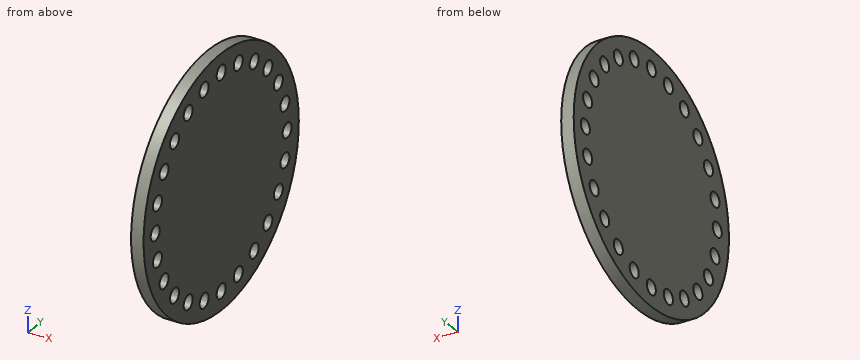
from build123d import *

# Parameters (mm, degrees)
F0_R     = 30
F0_R_2   = 1.75
F1_DEPTH = 3


with BuildPart() as f1:
    # F0 (on Right) → F1 (new body)
    with BuildSketch(Plane.YZ):
        Circle(F0_R)
        with Locations((-18.031223, -18.031223)):
            Circle(F0_R_2, mode=Mode.SUBTRACT)
        with Locations((-6.599886, -24.631109)):
            Circle(F0_R_2, mode=Mode.SUBTRACT)
        with Locations((-12.75, -22.083648)):
            Circle(F0_R_2, mode=Mode.SUBTRACT)
        with Locations((-22.083648, -12.75)):
            Circle(F0_R_2, mode=Mode.SUBTRACT)
        with Locations((-24.631109, -6.599886)):
            Circle(F0_R_2, mode=Mode.SUBTRACT)
        with Locations((0, -25.5)):
            Circle(F0_R_2, mode=Mode.SUBTRACT)
        with Locations((6.599886, -24.631109)):
            Circle(F0_R_2, mode=Mode.SUBTRACT)
        with Locations((12.75, -22.083648)):
            Circle(F0_R_2, mode=Mode.SUBTRACT)
        with Locations((18.031223, -18.031223)):
            Circle(F0_R_2, mode=Mode.SUBTRACT)
        with Locations((22.083648, -12.75)):
            Circle(F0_R_2, mode=Mode.SUBTRACT)
        with Locations((24.631109, -6.599886)):
            Circle(F0_R_2, mode=Mode.SUBTRACT)
        with Locations((-25.5, 0)):
            Circle(F0_R_2, mode=Mode.SUBTRACT)
        with Locations((-24.631109, 6.599886)):
            Circle(F0_R_2, mode=Mode.SUBTRACT)
        with Locations((-22.083648, 12.75)):
            Circle(F0_R_2, mode=Mode.SUBTRACT)
        with Locations((-18.031223, 18.031223)):
            Circle(F0_R_2, mode=Mode.SUBTRACT)
        with Locations((-12.75, 22.083648)):
            Circle(F0_R_2, mode=Mode.SUBTRACT)
        with Locations((-6.599886, 24.631109)):
            Circle(F0_R_2, mode=Mode.SUBTRACT)
        with Locations((25.5, 0)):
            Circle(F0_R_2, mode=Mode.SUBTRACT)
        with Locations((24.631109, 6.599886)):
            Circle(F0_R_2, mode=Mode.SUBTRACT)
        with Locations((22.083648, 12.75)):
            Circle(F0_R_2, mode=Mode.SUBTRACT)
        with Locations((12.75, 22.083648)):
            Circle(F0_R_2, mode=Mode.SUBTRACT)
        with Locations((0, 25.5)):
            Circle(F0_R_2, mode=Mode.SUBTRACT)
        with Locations((6.599886, 24.631109)):
            Circle(F0_R_2, mode=Mode.SUBTRACT)
        with Locations((18.031223, 18.031223)):
            Circle(F0_R_2, mode=Mode.SUBTRACT)
    extrude(amount=F1_DEPTH)


solid = f1.part
Check sheet for the modelled part. Datum: model origin and axes. Units: mm. Coordinates: 2 decimals unless noted, no trailing zeros. Loops run counter-clockwise (first coordinate to the right, second up) from the corner with the lowest first, then second, coordinate; pieces in that order, holes last. Notation, with made-up numbers: (22.25, 60) -> (73.25, 60) arc R17 ccw to (73.25, 93) -> close; hole circle Ø4 at (26, -7). An arc over 180 degrees is marked (long way). Answer in a Markdown table with one row per item.
1. Material ranges on line 1 along Z through (x, y) = (1.5, 0); line 2 along Y through (x, z) = (0.35, 12); line 3 along Y through (x, z) = (0.95, -24), recorded low to high. Write a range as [from, to].
Check values:
| item | result |
|---|---|
| line 1 | z = [-30, -27.25], [-23.75, 23.75], [27.25, 30] |
| line 2 | y = [-27.5, -23.66], [-20.5, 20.5], [23.66, 27.5] |
| line 3 | y = [-18, -8.23], [-4.97, -0.9], [0.9, 4.97], [8.23, 18] |
2. Sectioned sample at A-A, the plane z = 0. Record the boundary of the cut face in (x, y), then the cut area to 3 significant figures.
Check values:
| item | result |
|---|---|
| outline | (0, -30) -> (3, -30) -> (3, -27.25) -> (0, -27.25) -> close; (0, -23.75) -> (3, -23.75) -> (3, 23.75) -> (0, 23.75) -> close; (0, 27.25) -> (3, 27.25) -> (3, 30) -> (0, 30) -> close |
| area | 159 mm2 |
3. Sectioned sample at D-D, the plane y = -25.5. Record the boundary of the cut face in (x, z), then the cut area to 3 significant figures.
Check values:
| item | result |
|---|---|
| outline | (0, -15.8) -> (3, -15.8) -> (3, -8.12) -> (0, -8.12) -> close; (0, -5.08) -> (3, -5.08) -> (3, -1.75) -> (0, -1.75) -> close; (0, 1.75) -> (3, 1.75) -> (3, 5.08) -> (0, 5.08) -> close; (0, 8.12) -> (3, 8.12) -> (3, 15.8) -> (0, 15.8) -> close |
| area | 66.1 mm2 |
4. Sectioned sample at C-C, the plane x = 1.95. Give the number of separate pieces and of enclosed holes in the cut face, then the cut area to 3 significant figures.
Check values:
| item | result |
|---|---|
| separate pieces | 1 |
| enclosed holes | 24 |
| area | 2,600 mm2 |
5. Go/stop test with flat-tipped pins: pin 1 (1 mm diameter, centred on x = 1.5, y = 16, fed in from +Z); pin 2 (3 mm diameter, centred on y = -18.03, z = -18.03, fed in from +X); pin 3 (1 mm diameter, centred on x = 2, y = 20.5, fed in from -Z). Record where each tip stops, or that it passes through.
Check values:
| item | result |
|---|---|
| pin 1 | stops at z = 25.69 |
| pin 2 | passes through |
| pin 3 | stops at z = -22.36 |
